For this review, use the dimensioned drawing (mm, ordinates from the lowest corner) and the shaded views. Coordinates: 2 decimals unless noted, no trailing zeros. Order: outer loops, then holes, each group sorted by start corner. A loop starts at its lowest first (then second) coordinate and runs counter-clockwise, first axis right, second up. Notation, with made-up numbers: M 58.25,15 L 75.25,15 A20 ccw 75.25,32 Z; hole C 70,19.25 d5. An arc over 180 degrees is marked long. Answer in a Markdown table with one row per item.
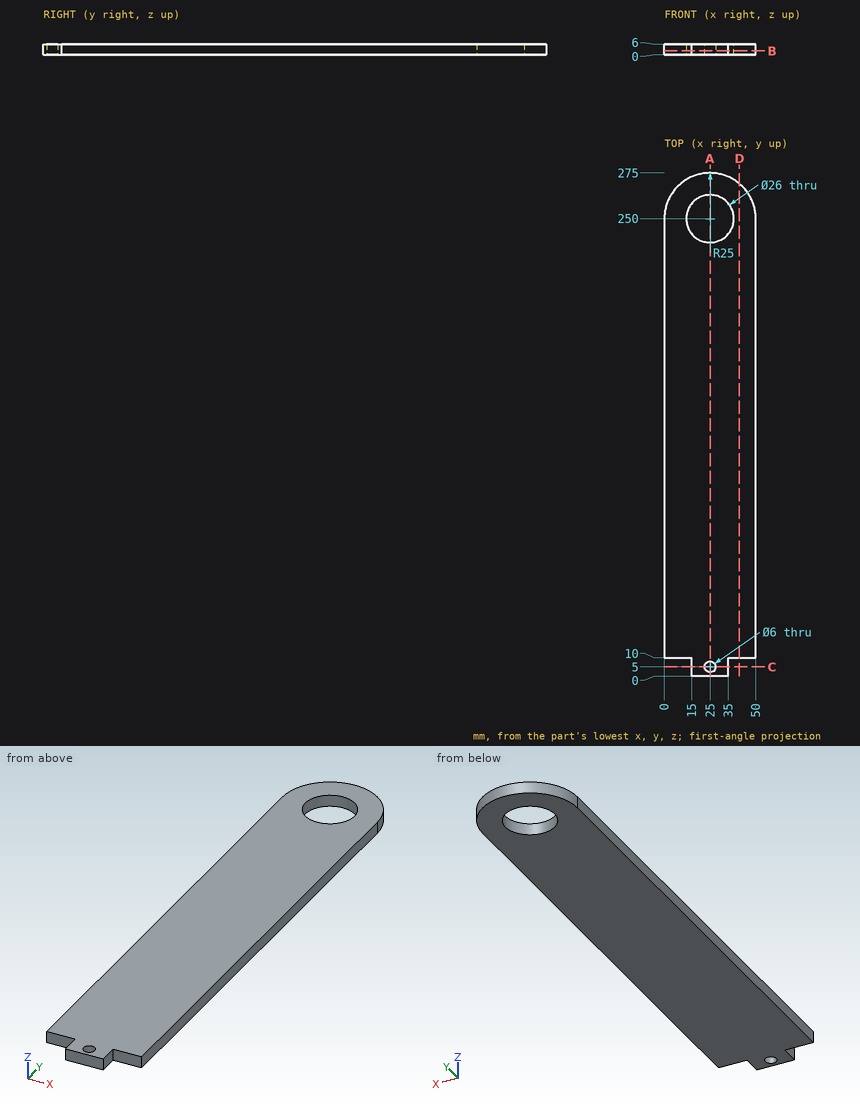
(1) Take a section at D-D (x = 41). Write out the cut boundary in (y, z).
Report:
| item | result |
|---|---|
| outline | M 10,0 L 269.21,0 L 269.21,6 L 10,6 Z |
(2) Take a section at B-B (z = 2.2). Write out the cut boundary in (x, y).
Report:
| item | result |
|---|---|
| outline | M 0,10 L 15,10 L 15,0 L 35,0 L 35,10 L 50,10 L 50,250 A25 ccw 0,250 Z; hole C 25,250 d26; hole C 25,5 d6 |
(3) To check wall thickness, follow line 1 (Y direction, x = 25, z = 3.85); line 2 (X direction, y = 5, z = 2.4); line 3 (Y direction, x = 28.5, z = 1.5). State the ranges of each line that lie inside material, in increasing order. Write a range as [from, to].
Report:
| item | result |
|---|---|
| line 1 | [0, 2], [8, 237], [263, 275] |
| line 2 | [15, 22], [28, 35] |
| line 3 | [0, 237.48], [262.52, 274.75] |
(4) Take a section at C-C (y = 5). Write out the cut boundary in (x, z), then the cut area to 3 significant figures.
Report:
| item | result |
|---|---|
| outline | M 15,0 L 22,0 L 22,6 L 15,6 Z; M 28,0 L 35,0 L 35,6 L 28,6 Z |
| area | 84.0 mm^2 |
(5) Insertion check: P1, Ø3, axis at x = 6.5, z = 4, coming from the -Y side; P2, Ø2, axis at x = 16, z = 3, coming from the +Y side. Each pin has a flat end and moves straight along its axis. Give the tip position at first contact, or say it passes through.
Report:
| item | result |
|---|---|
| P1 | y = 10 |
| P2 | y = 273.69 |
(6) Take a section at A-A (x = 25). Write out the cut boundary in (y, z), then the cut area to 3 significant figures.
Report:
| item | result |
|---|---|
| outline | M 0,0 L 2,0 L 2,6 L 0,6 Z; M 8,0 L 237,0 L 237,6 L 8,6 Z; M 263,0 L 275,0 L 275,6 L 263,6 Z |
| area | 1,460 mm^2 |
